Check sheet for the drawn part. Datum: minimum x, y, z corner. Units: mm. A direction names the side the tool comes from. Give positions to 0.01 mm unless a question says otherwise; leave off trailing zeros. Write each loop counter-clockwise with the first axis right and the second up, starting at its lowest first coordinate (ties: lowest second). Pieces come first, ordered by that corner, then holes. Notation, with made-up numbers: (62, 62.25) -> (86, 62.25) arc R19 cw to (86, 78.25) -> close; hole circle Ø7 at (2, 31.25). An arc over 180 degrees is marked (long way). Write item = value, one per line. Start each with the question number.
1. Cross-section at D-D, the plane y = 7.5. Record the cut outline in (x, z).
2. Mould release check, pull along Z, two halves, no side actions. Record for the marked faces 3, 4 and 5: pulls with the +Z half, pulls with the -Z half, needs draft (parallel to the pull), parting line crosses it, or undercut.
3. Cross-section at B-B, the plane z = 4. Record the cut outline in (x, y).
4. Cross-section at A-A, the plane y = 10.5. Record the cut outline in (x, z), plus the area to 3 significant figures.
5. Set-up check for the marked faces 1 and 2: record each of +Z, -Z, +X, -X, +Y, -Y from which the full face is reachable in a straight line by a thin tool's end or side.
6. Cross-section at C-C, the plane x = 3.2. Record the cut outline in (y, z) (1 decimal).
7. Thickness scan on line 1 along Y through (x, z) = (4, 2.25); line 2 along Y through (x, z) = (1.45, 3.25); line 3 along X through (y, z) = (10.5, 2.25) (1 decimal). Record the ranges inside material, lowest first.
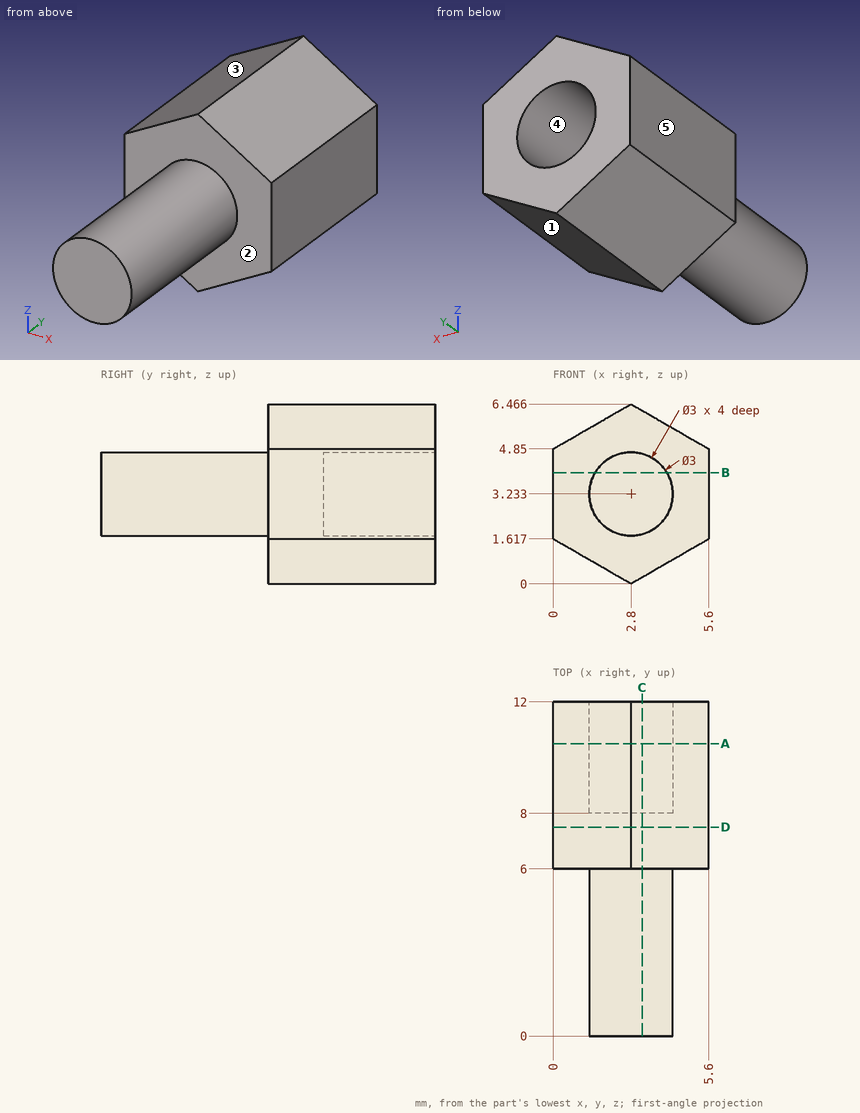
Answers:
q1.outline = (0, 1.62) -> (2.8, 0) -> (5.6, 1.62) -> (5.6, 4.85) -> (2.8, 6.47) -> (0, 4.85) -> close
q2.face_3 = pulls with the +Z half
q2.face_4 = undercut
q2.face_5 = needs draft
q3.outline = (0, 6) -> (1.51, 6) -> (1.51, 0) -> (4.09, 0) -> (4.09, 6) -> (5.6, 6) -> (5.6, 12) -> (4.09, 12) -> (4.09, 8) -> (1.51, 8) -> (1.51, 12) -> (0, 12) -> close
q4.outline = (0, 1.62) -> (2.8, 0) -> (5.6, 1.62) -> (5.6, 4.85) -> (2.8, 6.47) -> (0, 4.85) -> close; hole circle Ø3 at (2.8, 3.23)
q4.area = 20.1 mm^2
q5.face_1 = -Z, +X, +Y, -Y
q5.face_2 = -Y
q6.outline = (0, 1.8) -> (6, 1.8) -> (6, 0.2) -> (12, 0.2) -> (12, 1.8) -> (8, 1.8) -> (8, 4.7) -> (12, 4.7) -> (12, 6.2) -> (6, 6.2) -> (6, 4.7) -> (0, 4.7) -> close
q7.line_1 = 6 to 12
q7.line_2 = 0 to 8
q7.line_3 = 0 to 1.7, 3.9 to 5.6
